Read the model definition and answer for the solid it produces. Units are mm, in the model's axes. Face numbers are marked on the shaded views. Coordinates: 2 decimals unless noted, no trailing zeros. Loops run counter-clockwise (first coordinate to the right, second up) from the corner with the lowest first, then second, coordinate; pieces in that order, holes last.
Q1. A flat-ended cylindrical pin translates along its axis: P1, Ø3, axis at x = -15, y = -1.5, coming from the +Z side. Find the tip coordinate at first contact, or state that the pin passes through.
Q2. Section B-B (z = 0) is taken. Give the vertices of the cut face in (x, y).
Q3. Straight lines are drawn through the part: line 1 (X direction, y = 0, z = 1.75); line 2 (Y direction, x = -21, z = 2); line 3 (X direction, y = -1, z = 3.5). For each, find the intervals that lie inside material, in ascending order.
Q4. The mould has two halves that part along Y. Classify the marked faces 1, 2 and 3: pulls with the +Y half, pulls with the -Y half, needs draft (parallel to the pull), parting line crosses it, or undercut.
Q5. Section A-A (y = 0) is taken. Give the vertices of the cut face in (x, z).
Q6. Section D-D (y = -2) is taken. Give the vertices of the cut face in (x, z), then the cut area to 3 significant figures.
Q7. Section C-C (x = -21) is taken. Give the vertices of the cut face in (y, z).
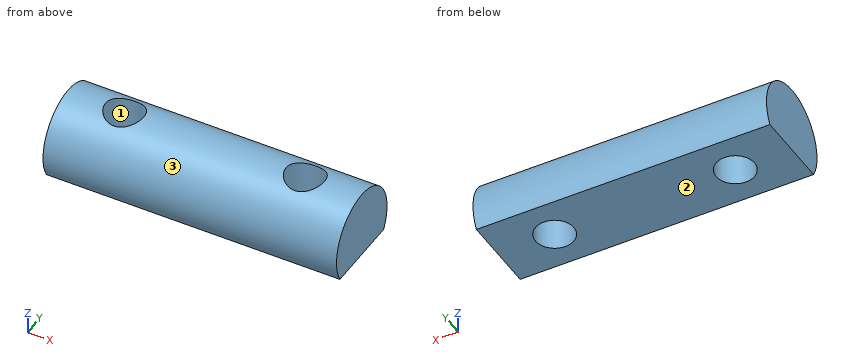
from build123d import *

# Parameters (mm, degrees)
SKETCH_R        = 4
PAD_DEPTH       = 26
SKETCH001_W     = 4
SKETCH001_H     = 12
POCKET_DEPTH    = 26
SKETCH002_R     = 1.7
POCKET001_DEPTH = 7


with BuildPart() as part:
    # Sketch → Pad (new body)
    with BuildSketch(Plane.ZY):
        Circle(SKETCH_R)
    extrude(amount=PAD_DEPTH)

    # Sketch001 → Pocket (cut)
    with BuildSketch(Plane.ZY.offset(26)):
        with Locations((-4, -1)):
            Rectangle(SKETCH001_W, SKETCH001_H)
    extrude(amount=-POCKET_DEPTH, mode=Mode.SUBTRACT)

    # Sketch002 → Pocket001 (cut)
    with BuildSketch(Plane(origin=(0, 0, -2), x_dir=(0, -1, 0), z_dir=(0, 0, -1))):
        with Locations((0, 21)):
            Circle(SKETCH002_R)
        with Locations((0, 5)):
            Circle(SKETCH002_R)
    extrude(amount=-POCKET001_DEPTH, mode=Mode.SUBTRACT)


solid = part.part
Numbers:
1. P1: stops at z = 4
2. outline: (-26, -4) - (0, -4) - (0, 4) - (-26, 4) - close; hole circle Ø3.4 at (-21, 0); hole circle Ø3.4 at (-5, 0)
3. line 1: x = -26 to -22.7, -19.3 to -6.7, -3.3 to 0
3. line 2: y = -3.46 to -1.7, 1.7 to 3.46
3. line 3: x = -26 to -22.37, -19.63 to -6.37, -3.63 to 0
4. face 1: undercut
4. face 2: needs draft
4. face 3: parting line crosses it
5. outline: (-26, -2) - (-22.7, -2) - (-22.7, 4) - (-26, 4) - close; (-19.3, -2) - (-6.7, -2) - (-6.7, 4) - (-19.3, 4) - close; (-3.3, -2) - (0, -2) - (0, 4) - (-3.3, 4) - close
6. outline: (-26, -2) - (0, -2) - (0, 3.46) - (-26, 3.46) - close
6. area: 142 mm2
7. outline: (-3.46, -2) - (-1.7, -2) - (-1.7, 3.62) arc R4 ccw to start; (1.7, -2) - (3.46, -2) arc R4 ccw to (1.7, 3.62) - close
